Verification items for the finished model (mm, model axes). Face numbers are marked on the shaded views. A direction names the side the tool comes from. Coordinates: 2 decimals unless noted, no trailing zeros. Order: outer loops, then holes, each group sorted by start corner. A loop starts at its lowest first (then second) coordinate and runs counter-clockwise, first axis right, second up. Notation, with made-up numbers: (5, 68.25) -> (62, 68.25) arc R21 ccw to (62, 84.25) -> close; hole circle Ø2 at (-31, -3.75). An arc over 180 degrees is marked (long way). Write item = value, one per line. Start each with the question number.
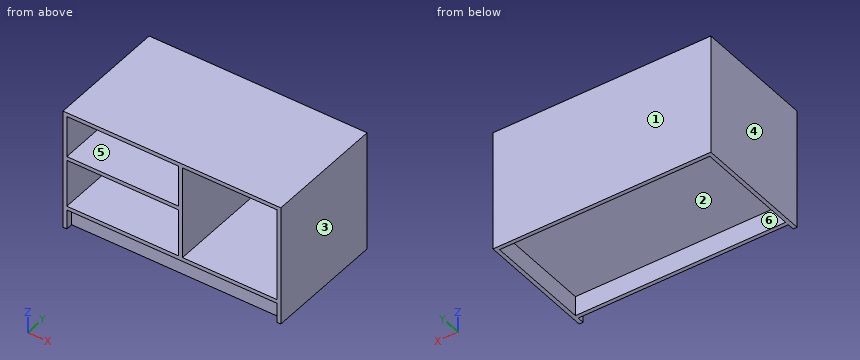
from build123d import *

# Parameters (mm, degrees)
F0_W      = 460.375
F0_H      = 15.875
F1_DEPTH  = 496.8875
F2_START  = -27.94
F0_W_2    = 865.1875
F0_H_2    = 81.28
F2_DEPTH  = 15.875
F3_START  = 437.1975
F2_FACE_W = 865.1875
F2_FACE_H = 81.28
F3_DEPTH  = 15.875
F4_START  = -495.3
F0_H_3    = 196.5325
F0_W_3    = 388.9375
F0_H_4    = 383.8575
F0_H_5    = 171.45
F4_DEPTH  = 1.5875


with BuildPart() as f1:
    # F0 (on Front) → F1 (new body)
    with BuildSketch(Plane.XZ):
        Polygon((881.0625, 0), (15.875, 0), (15.875, -15.875), (476.25, -15.875), (492.125, -15.875), (881.0625, -15.875), align=None)
        Polygon((896.9375, 0), (881.0625, 0), (881.0625, -15.875), (881.0625, -399.7325), (881.0625, -415.6075), (881.0625, -496.8875), (896.9375, -496.8875), align=None)
        Polygon((15.875, 0), (0, 0), (0, -496.8875), (15.875, -496.8875), (15.875, -415.6075), (15.875, -399.7325), (15.875, -203.2), (15.875, -187.325), (15.875, -15.875), align=None)
        with Locations((246.0625, -195.2625)):
            Rectangle(F0_W, F0_H)
        Polygon((492.125, -15.875), (476.25, -15.875), (476.25, -187.325), (476.25, -203.2), (476.25, -399.7325), (492.125, -399.7325), align=None)
        Polygon((15.875, -399.7325), (15.875, -415.6075), (881.0625, -415.6075), (881.0625, -399.7325), (492.125, -399.7325), (476.25, -399.7325), align=None)
    extrude(amount=-F1_DEPTH)

    # F0 (on Front) → F2 (join)
    with BuildSketch(Plane.XZ.offset(F2_START)):
        with Locations((448.46875, -456.2475)):
            Rectangle(F0_W_2, F0_H_2)
    extrude(amount=-F2_DEPTH)

    # F2_face (on face) → F3 (join)
    with BuildSketch(Plane(origin=(448.46875, 43.815, -456.2475), x_dir=(1, 0, 0), z_dir=(0, 1, 0)).offset(F3_START)):
        Rectangle(F2_FACE_W, F2_FACE_H)
    extrude(amount=F3_DEPTH)

    # F0 (on Front) → F4 (join)
    with BuildSketch(Plane.XZ.offset(F4_START)):
        with Locations((448.46875, -456.2475)):
            Rectangle(F0_W_2, F0_H_2)
        Polygon((15.875, -399.7325), (15.875, -415.6075), (881.0625, -415.6075), (881.0625, -399.7325), (492.125, -399.7325), (476.25, -399.7325), align=None)
        with Locations((246.0625, -301.46625)):
            Rectangle(F0_W, F0_H_3)
        with Locations((686.59375, -207.80375)):
            Rectangle(F0_W_3, F0_H_4)
        with Locations((246.0625, -195.2625)):
            Rectangle(F0_W, F0_H)
        Polygon((492.125, -15.875), (476.25, -15.875), (476.25, -187.325), (476.25, -203.2), (476.25, -399.7325), (492.125, -399.7325), align=None)
        with Locations((246.0625, -101.6)):
            Rectangle(F0_W, F0_H_5)
        Polygon((881.0625, 0), (15.875, 0), (15.875, -15.875), (476.25, -15.875), (492.125, -15.875), (881.0625, -15.875), align=None)
        Polygon((896.9375, 0), (881.0625, 0), (881.0625, -15.875), (881.0625, -399.7325), (881.0625, -415.6075), (881.0625, -496.8875), (896.9375, -496.8875), align=None)
        Polygon((15.875, 0), (0, 0), (0, -496.8875), (15.875, -496.8875), (15.875, -415.6075), (15.875, -399.7325), (15.875, -203.2), (15.875, -187.325), (15.875, -15.875), align=None)
    extrude(amount=-F4_DEPTH)


solid = f1.part
Item 1: Section check A-A (z = -425.5). Record the boundary of the cut face in (x, y) (1 decimal), then the cut area to 3 significant figures.
Item 2: Mould release check, pull along Y, two halves, no side actions. Record for the marked faces 1, 2 and 3: pulls with the +Y half, pulls with the -Y half, needs draft (parallel to the pull), parting line crosses it, or undercut.
Item 3: Thickness scan on line 1 (Z direction, x = 231, y = 269.5) (1 decimal); line 2 (Z direction, x = 175.5, y = 29.5) (1 decimal); line 3 (Z direction, x = 858, y = 383.5) (1 decimal). Record the ranges inside material, lowest first.
Item 4: Section check C-C (x = 655). Record the boundary of the cut face in (y, z) (1 decimal).
Item 5: Gauge pin test, flat ends, axial feed: P1, Ø22.5, axis at x = 501.5, y = 12, coming from the -Z side; P2, Ø10, axis at x = 505, z = -351.5, coming from the -Y side. Record the tip position at first contact, or that the pin passes through.
Item 6: Section check B-B (y = 129). State how many separate pieces and enclosed holes the cut face has, then the cut area to 3 significant figures.
Item 7: Tool access check on the marked faces 4, 5 and 6. Record the directions out of +Z, -Z, +X, -X, +Y, -Y that give a thin tool (end or side, any length) a straight path to the whole face; none if there is none.
Filled sheet:
q1.outline = (0, 0) -> (15.9, 0) -> (15.9, 27.9) -> (881.1, 27.9) -> (881.1, 0) -> (896.9, 0) -> (896.9, 496.9) -> (0, 496.9) -> close; hole (15.9, 43.8) -> (881.1, 43.8) -> (881.1, 481) -> (15.9, 481) -> close
q1.area = 43,200 mm^2
q2.face_1 = pulls with the +Y half
q2.face_2 = undercut
q2.face_3 = needs draft
q3.line_1 = -415.6 to -399.7, -203.2 to -187.3, -15.9 to 0
q3.line_2 = -496.9 to -399.7, -203.2 to -187.3, -15.9 to 0
q3.line_3 = -415.6 to -399.7, -15.9 to 0
q4.outline = (0, -415.6) -> (27.9, -415.6) -> (27.9, -496.9) -> (43.8, -496.9) -> (43.8, -415.6) -> (481, -415.6) -> (481, -496.9) -> (496.9, -496.9) -> (496.9, 0) -> (0, 0) -> (0, -15.9) -> (495.3, -15.9) -> (495.3, -399.7) -> (0, -399.7) -> close
q5.P1 = -415.61
q5.P2 = 495.3
q6.separate_pieces = 1
q6.enclosed_holes = 3
q6.area = 56,600 mm^2
q7.face_4 = +Z, -Z, -X, +Y, -Y
q7.face_5 = -Y
q7.face_6 = -Z
